Autodesk Inventor part; units mm, degrees
ref_plane "YZ Plane" through (0, 0, 0) normal (1, 0, 0) x (0, 1, 0)
ref_plane "XZ Plane" through (0, 0, 0) normal (0, 1, 0) x (-1, 0, 0)
ref_plane "XY Plane" through (0, 0, 0) normal (0, 0, 1) x (1, 0, 0)
sketch "Sketch1" plane through (0, 0, 0) normal (0, 0, 1) x (1, 0, 0)
  line L0 (0, 0) -> (10, 0)
  line L1 (10, 0) -> (10, 20)
  line L2 (10, 20) -> (0, 20)
  line L3 (0, 20) -> (0, 0)
  dimension "d0" = 10
  dimension "d1" = 20
extrude "Extrusion1" add sketch "Sketch1" along normal blind 6.5
sketch "Sketch2" plane through (0, 0, 6.5) normal (0, 0, 1) x (1, 0, 0)
  circle A0 centre (3, 15) radius 1.25
  circle A1 centre (3, 5) radius 1.25
  line L0 (10, 0) -> (10, 20)
  line L1 (10, 20) -> (0, 20)
  line L2 (0, 20) -> (0, 0)
  line L3 (0, 0) -> (10, 0)
  dimension "d4" = 5
  dimension "d5" = 2.5
  dimension "d6" = 3
  dimension "d7" = 5
  dimension "d8" = 3
  dimension "d9" = 2.5
extrude "Extrusion2" cut sketch "Sketch2" against normal through all contours A0 | A1
ref_plane "Work Plane1" through (0, 0, 3.25) normal (0, 0, 1) x (1, 0, 0)
properties part number "micro-switch"
Input: part model. Units: mm. Frame: model coordinates. Give positions to 0.01 mm unless a question says otherwise; leave off trailing zeros. Order: outer loops, then holes, each group sorted by start corner. A loop starts at its lowest first (then second) coordinate and runs counter-clockwise, first axis right, second up. Notation, with made-up numbers: (81, 17) -> (96, 17) arc R7 ccw to (96, 21) -> close; hole circle Ø11 at (88, -26.5). An arc over 180 degrees is marked (long way). Write each question's results on one line, items separated by ' | '. Start each with the question number.
Item 1: Line query: line 1 (Y direction, x = 3, z = 4); line 2 (Y direction, x = 2, z = 0.75). Output: solid intervals per line, ascending.
Item 2: Mould query, pull axis X, two halves, no side actions, for faces 1 (the cylindrical face through (3.577, 3.891, 3.296)), 2 (the flat face through (5, 0, 3)), 3 (the flat face through (10, 10, 3)). Classes: pulls with the +X half, pulls with the -X half, needs draft (parallel to the pull), parting line crosses it, or undercut.
Item 3: Cut plane B-B on x = 3. Return the cut outline in (y, z).
Item 4: Cut plane A-A on y = 5.75. Return the cut outline in (x, z), then the cut area to 3 significant figures.
Item 5: Cut plane C-C on z = 6. Return the cut outline in (x, y), then the cut area to 3 significant figures.
Item 6: Cut plane D-D on y = 14.75. Return the cut outline in (x, z), then the cut area to 3 significant figures.
Established:
1) line 1: 0 to 3.75, 6.25 to 13.75, 16.25 to 20 | line 2: 0 to 4.25, 5.75 to 14.25, 15.75 to 20
2) face 1: undercut | face 2: needs draft | face 3: pulls with the +X half
3) outline: (0, 0) -> (3.75, 0) -> (3.75, 6.5) -> (0, 6.5) -> close; (6.25, 0) -> (13.75, 0) -> (13.75, 6.5) -> (6.25, 6.5) -> close; (16.25, 0) -> (20, 0) -> (20, 6.5) -> (16.25, 6.5) -> close
4) outline: (0, 0) -> (2, 0) -> (2, 6.5) -> (0, 6.5) -> close; (4, 0) -> (10, 0) -> (10, 6.5) -> (4, 6.5) -> close | area: 52.0 mm^2
5) outline: (0, 0) -> (10, 0) -> (10, 20) -> (0, 20) -> close; hole circle Ø2.5 at (3, 5); hole circle Ø2.5 at (3, 15) | area: 190 mm^2
6) outline: (0, 0) -> (1.78, 0) -> (1.78, 6.5) -> (0, 6.5) -> close; (4.22, 0) -> (10, 0) -> (10, 6.5) -> (4.22, 6.5) -> close | area: 49.1 mm^2
